from build123d import *

# Parameters (mm, degrees)
EXTRUDE_1_DEPTH     = 531
SKETCH_2_W          = 23
SKETCH_2_H          = 23
CUT_EXTRUDE_1_DEPTH = 26


with BuildPart() as part:
    # Эскиз1 → Вытянуть-Тонкостенный1 (new body)
    with BuildSketch(Plane(origin=(0, 0, 0), x_dir=(0, 0, -1), z_dir=(1, 0, 0))):
        Polygon((0, 25), (0, 0), (25, 0), (25, 2), (2, 2), (2, 25), align=None)
    extrude(amount=EXTRUDE_1_DEPTH)

    # Эскиз2 → Вырез-Вытянуть1 (cut, through all)
    with BuildSketch(Plane.XZ):
        with Locations((11.5, -13.5)):
            Rectangle(SKETCH_2_W, SKETCH_2_H)
        with Locations((519.5, -13.5)):
            Rectangle(SKETCH_2_W, SKETCH_2_H)
    extrude(amount=-CUT_EXTRUDE_1_DEPTH, mode=Mode.SUBTRACT)


solid = part.part
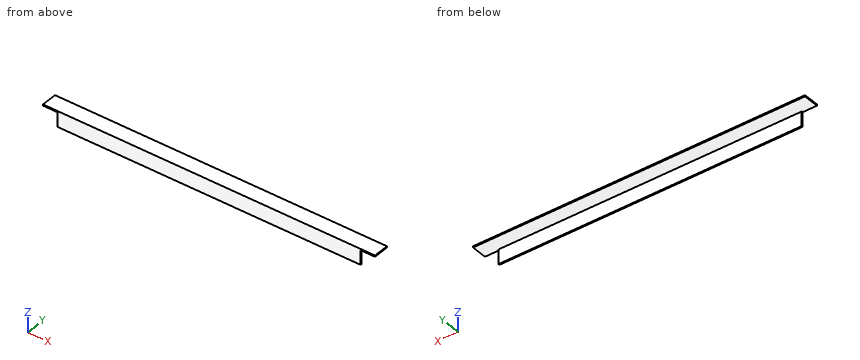
Geometry: final body of the model. Coordinates: model frame, mm. Coordinates: 2 decimals unless noted, no trailing zeros. Order: outer loops, then holes, each group sorted by start corner. A loop starts at its lowest first (then second) coordinate and runs counter-clockwise, first axis right, second up. Notation, with made-up numbers: (13, 82) - (55, 82) arc R30 ccw to (55, 113) - close; hole circle Ø9 at (1.25, 28). An arc over 180 degrees is marked (long way). Use one line per item in the form item = value.
1) Pin query (flat end, axial travel): pin 1 (6 mm diameter, centred on x = 116.5, y = 16, fed in from -Z); pin 2 (10 mm diameter, centred on x = 60, z = -20.5, fed in from +Y); pin 3 (2 mm diameter, centred on y = 1, z = -11.5, fed in from +X). Return the tip coordinate at first contact, or that it passes through.
Solutions:
pin_1 = -2
pin_2 = 2
pin_3 = 508
2) Ray query, L1, parallel to Z at x = 415, y = 12.5; L2, parallel to Y at x = 263, z = -6. Return the intervals inside material, ascending.
Solutions:
L1 = -2 to 0
L2 = 0 to 2
3) Section C-C (z = -9.5). Return loops of the section in (x, y).
Solutions:
outline = (23, 0) - (508, 0) - (508, 2) - (23, 2) - close
4) Section A-A (x = 113). Return loops of the section in (y, z), then the cut area to 3 significant figures.
Solutions:
outline = (0, -25) - (2, -25) - (2, -2) - (25, -2) - (25, 0) - (0, 0) - close
area = 96.0 mm^2
5) Section B-B (y = 16.5). Return loops of the section in (x, z), then the cut area to 3 significant figures.
Solutions:
outline = (0, -2) - (531, -2) - (531, 0) - (0, 0) - close
area = 1,060 mm^2
